Here's how the part is built. I have some questions about the finished solid (model axes, mm). A direction names the side the tool comes from. Round coordinates to 2 decimals unless told otherwise and drop trailing zeros. Loops run counter-clockwise (first coordinate to the right, second up) from the corner with the lowest first, then second, coordinate; pieces in that order, holes last. Notation, with made-up numbers: (-10.5, 33) - (32.5, 33) arc R8 ccw to (32.5, 45) - close; hole circle Ø3 at (3, -31.5). An arc over 180 degrees is marked (long way). Answer as a JSON object with one key per item and string values. Group by question number.
1) Will these pins go through, and if not, where does the flat tip stop? P1, Ø1.1, axis at x = -0.5, y = 171, coming from the +Z side (3 decimals); P2, Ø5, axis at y = 110.5, z = 7.5, coming from the -X side; P3, Ø10, axis at x = -10.5, y = 30, coming from the +Z side.
2) I want a section at B-B, the plane y = 171.45. Please give me the cut outline in (x, z) (3 decimals).
3) Which directions (+Z, -Z, +X, -X, +Y, -Y) give clear straight access to the entire face, cutting with the end or side of a thin tool? Please do faces 4 (the face through (-1.51, 170.29, -14.19)), 5 (the face through (0, 171, 13.865)), 6 (the face through (0, 186.69, 0)).
4) I want a section at A-A, the plane y = 118. Please give me the cut outline in (x, z), then the cut area to 3 significant figures.
5) If I drill on line 1 along Z through (x, y) = (1, 137); line 2 along Y through (x, z) = (8.5, -5); line 3 along Y through (x, z) = (0, -14) (3 decimals), over which ranges is the centre line in solid material (lowest first)? Write a range as [from, to].
6) If we mould it in two halves opening along X, with no side actions, what happens to faces 1 (the face through (6.691, 89.534, 12.864)), 2 (the face through (-1.51, 170.29, 14.19)), 3 (the face through (0, 0, 0))? For each: pulls with the +X half, pulls with the -X half, needs draft (parallel to the pull), parting line crosses it, or undercut.
from build123d import *

# Parameters (mm, degrees)
SKETCH1_R           = 14.5
BOSS_EXTRUDE1_DEPTH = 186.69
FILLET1_R           = 5.08
SKETCH5_R           = 1.905
CUT_EXTRUDE4_DEPTH  = 0.635
SKETCH2_R           = 1.905
CUT_EXTRUDE5_DEPTH  = 0.635


with BuildPart() as part:
    # Sketch1 → Boss-Extrude1 (new body)
    with BuildSketch(Plane(origin=(0, 0, 0), x_dir=(1, 0, 0), z_dir=(0, 1, 0))):
        Circle(SKETCH1_R)
    extrude(amount=BOSS_EXTRUDE1_DEPTH)

    # Fillet1
    fillet1_edges = [part.edges().sort_by_distance(p)[0] for p in [
        (-14.5, 186.69, 0),
    ]]
    fillet(fillet1_edges, radius=FILLET1_R)

    # Sketch5 → Cut-Extrude4 (cut)
    with BuildSketch(Plane.XY.offset(-14.499999956)):
        with Locations((0, 171.45)):
            Circle(SKETCH5_R)
    extrude(amount=CUT_EXTRUDE4_DEPTH, mode=Mode.SUBTRACT)

    # Sketch2 → Cut-Extrude5 (cut)
    with BuildSketch(Plane.XY.offset(14.499999956)):
        with Locations((0, 171.45)):
            Circle(SKETCH2_R)
    extrude(amount=-CUT_EXTRUDE5_DEPTH, mode=Mode.SUBTRACT)


solid = part.part
Outcome:
{
 "1": {"P1": "z = 13.865", "P2": "x = -13.61", "P3": "z = 13.42"},
 "2": {"outline": "(-1.905, -14.374) - (-1.905, -13.865) - (1.905, -13.865) - (1.905, -14.374) arc R14.5 ccw to (1.905, 14.374) - (1.905, 13.865) - (-1.905, 13.865) - (-1.905, 14.374) arc R14.5 ccw to start"},
 "3": {"face 4": "-Z", "face 5": "+Z", "face 6": "+Z, -Z, +X, -X, +Y"},
 "4": {"outline": "circle Ø29 at (0, 0)", "area": "661 mm^2"},
 "5": {"line 1": "[-14.47, 14.47]", "line 2": "[0, 186.67]", "line 3": "[0, 169.545], [173.355, 183.808]"},
 "6": {"face 1": "parting line crosses it", "face 2": "undercut", "face 3": "needs draft"}
}
